```python
from build123d import *

# Parameters (mm, degrees)
SKETCH1_R           = 4.7625
BOSS_EXTRUDE1_DEPTH = 41.275
SKETCH2_W           = 0.7366
SKETCH2_H           = 2.54
CHAMFER1_SIZE       = 0.254


with BuildPart() as part:
    # Sketch1 → Boss-Extrude1 (new, symmetric)
    with BuildSketch(Plane.XY):
        Circle(SKETCH1_R)
    extrude(amount=BOSS_EXTRUDE1_DEPTH, both=True)

    # Sketch2 → Cut-Revolve1 (revolve, cut)
    with BuildSketch(Plane(origin=(0, 0, 0), x_dir=(0, 0, -1), z_dir=(1, 0, 0)), mode=Mode.PRIVATE) as cut_revolve1_sk:
        with Locations((-40.0558, 5.7404)):
            Rectangle(SKETCH2_W, SKETCH2_H)
    cut_revolve1 = revolve(cut_revolve1_sk.sketch.rotate(Axis((0, 0, 0), (0, 0, 1)), 90), axis=Axis((0, 0, 0), (0, 0, 1)), mode=Mode.SUBTRACT)

    # Chamfer1
    chamfer1_edges = [part.edges().sort_by_distance(p)[0] for p in [
        (-4.7625, 0, -41.275),
        (-4.7625, 0, 41.275),
    ]]
    chamfer(chamfer1_edges, length=CHAMFER1_SIZE)

    # Mirror3: Cut-Revolve1 across plane
    add(cut_revolve1.mirror(Plane.XY), mode=Mode.SUBTRACT)


solid = part.part
```
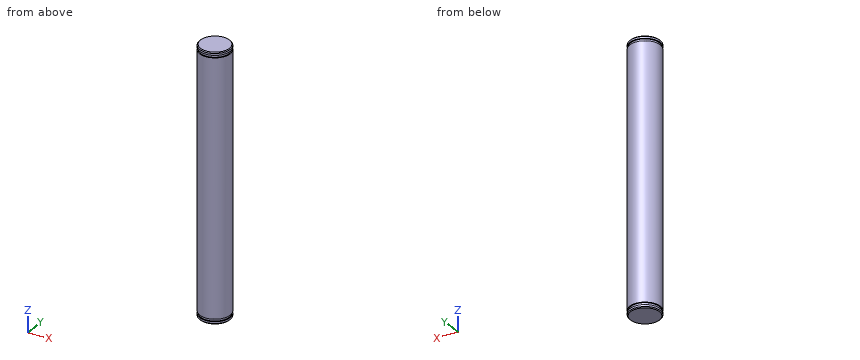
Work out the finished part from the listing and answer in its coordinate system (mm). Give positions to 0.01 mm unless a question says otherwise; leave off trailing zeros. Write each loop counter-clockwise with the first axis right and the second up, starting at its lowest first coordinate (ties: lowest second). Pieces come first, ordered by that corner, then holes. Notation, with made-up numbers: (29.25, -13.5) -> (55.25, -13.5) arc R20 ccw to (55.25, 1.5) -> close; hole circle Ø6 at (78.5, 50.25). An arc over 180 degrees is marked (long way). Write item = value, one per line.
Q1. Consider line 1 along Z through (x, y) = (3.75, -2.5) (1 decimal); line 2 along Z through (x, y) = (1, 4.5); line 3 along X through (y, z) = (1.5, 20). Determine where each line is inside the solid, lowest interval first.
Computed values:
line_1 = -41.3 to -40.4, -39.7 to 39.7, 40.4 to 41.3
line_2 = -41.17 to -40.42, -39.69 to 39.69, 40.42 to 41.17
line_3 = -4.52 to 4.52
Q2. Flat-ended cylindrical pins translate along their axes: pin 1 Ø4 at (x, z) = (-1.5, 21) entering from -Y; pin 2 Ø4 at (y, z) = (-3.5, 20.5) entering from +X; pin 3 Ø1 at (x, z) = (3.5, -30.5) entering from +Y; pin 4 Ø1 at (x, z) = (-1, -29) entering from +Y. Find the tip coordinate at first contact, or state that the pin passes through.
Computed values:
pin_1 = -4.76
pin_2 = 4.52
pin_3 = 3.7
pin_4 = 4.74
Q3. Section A-A on z = 5 is taken. Determine the outline of the cut face in (x, y) (1 decimal), and give its area (3 significant figures).
Computed values:
outline = circle Ø9.5 at (0, 0)
area = 71.3 mm^2
